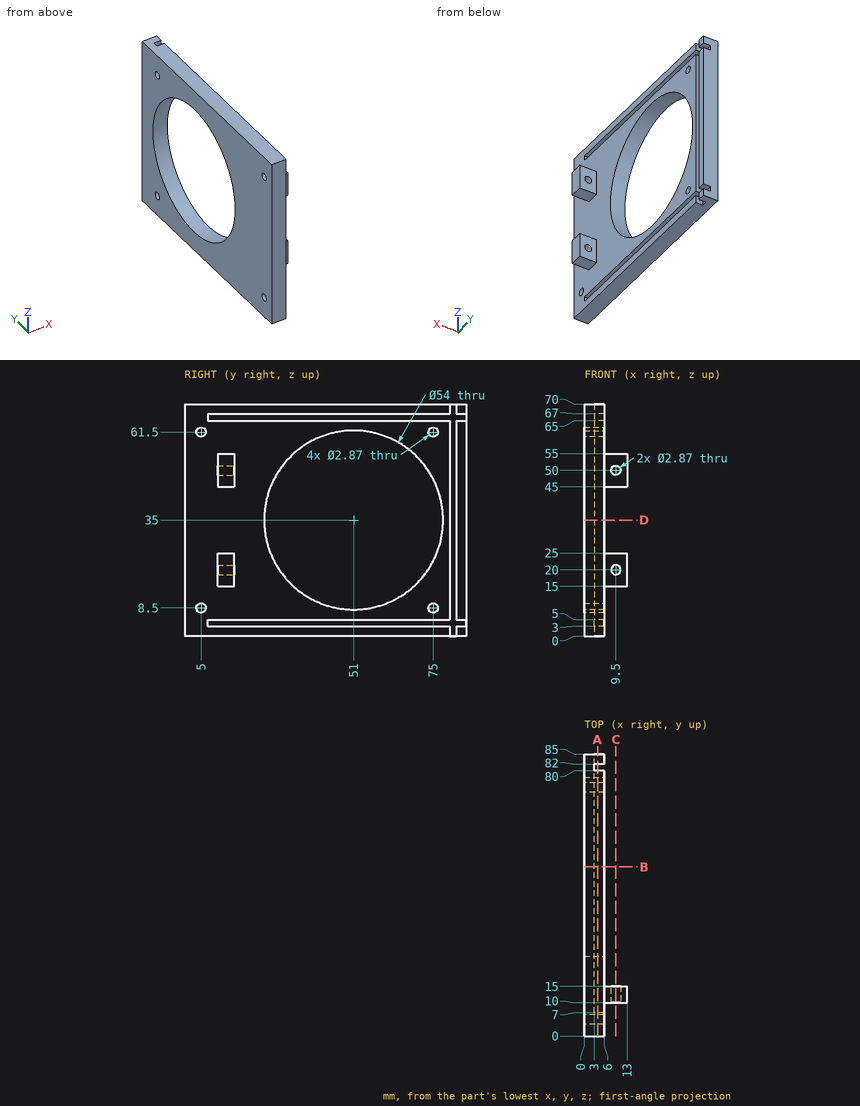
Design review of the part shown in the three views and the two pictorial views. Dimensions are in mm from the part's minimum x, y and z. Round coordinates to 2 decimals unless told otherwise and drop trailing zeros. Loops run counter-clockwise (first coordinate to the right, second up) from the corner with the lowest first, then second, coordinate; pieces in that order, holes last. Notation, with made-up numbers: (29.25, 10) -> (48.25, 10) arc R27 cw to (48.25, 33) -> close; hole circle Ø3 at (16.5, 60). An arc over 180 degrees is marked (long way). Answer as a JSON object with one key per item and string values. Group by question number.
1) We need section B-B on y = 51. Write out the cut boundary in (x, z), then the cut area to 3 significant figures.
2) We need section C-C on x = 9.5. Write out the cut boundary in (y, z) (3 decimals), then the cut area to 3 significant figures.
3) For line 1 (Z direction, x = 9.5, y = 11.3) (3 decimals); line 2 (Z direction, x = 3.45, y = 75) (3 decimals); line 3 (Y direction, x = 5.75, z = 38.5), list the stretches that pass through material, from the lowest coordinate up. Write a range as [from, to].
4) We need section D-D on z = 35. Write out the cut boundary in (x, y), then the cut area to 3 significant figures.
5) We need section A-A on x = 4. Give the number of separate pieces and of enclosed holes in the cut face, then the cut area to 3 significant figures.
6) For pin 1 Ø1 at (y, z) = (26.5, 15) entering from +X; pin 2 Ø4 at (x, y) = (7.5, 71.5) entering from -Z; pin 3 Ø1.5 at (x, z) = (11, 21) entering from -Y, all flat-tipped, find the tip position at first contact; note any pin that passes through.
Result set:
{
 "1": {"outline": "(0, 0) -> (6, 0) -> (6, 3) -> (3, 3) -> (3, 5) -> (6, 5) -> (6, 8) -> (0, 8) -> close; (0, 62) -> (6, 62) -> (6, 65) -> (3, 65) -> (3, 67) -> (6, 67) -> (6, 70) -> (0, 70) -> close", "area": "84.0 mm²"},
 "2": {"outline": "(10, 15) -> (15, 15) -> (15, 18.565) -> (10, 18.565) -> close; (10, 21.435) -> (15, 21.435) -> (15, 25) -> (10, 25) -> close; (10, 45) -> (15, 45) -> (15, 48.565) -> (10, 48.565) -> close; (10, 51.435) -> (15, 51.435) -> (15, 55) -> (10, 55) -> close", "area": "71.3 mm²"},
 "3": {"line 1": "[15, 18.565], [21.435, 25], [45, 48.565], [51.435, 55]", "line 2": "[0, 3], [5, 7.065], [9.935, 22.631], [47.369, 60.065], [62.935, 65], [67, 70]", "line 3": "[0, 24.23], [77.77, 80], [82, 85]"},
 "4": {"outline": "(0, 0) -> (6, 0) -> (6, 24) -> (0, 24) -> close; (0, 78) -> (6, 78) -> (6, 80) -> (3, 80) -> (3, 82) -> (6, 82) -> (6, 85) -> (0, 85) -> close", "area": "180 mm²"},
 "5": {"separate pieces": "4", "enclosed holes": "5", "area": "3,190 mm²"},
 "6": {"pin 1": "x = 6", "pin 2": "z = 0", "pin 3": "y = 10"}
}
